Here's the drawing with two shaded views (mm, measured from the low corner). I have some questions. A direction names the side the tool comes from. Round coordinates to 2 decimals unless told otherwise and drop trailing zeros. Loops run counter-clockwise (first coordinate to the right, second up) from the corner with the lowest first, then second, coordinate; pieces in that order, holes last. Notation, with made-up numbers: (71, 51.5) -> (87, 51.5) arc R25 cw to (87, 88.5) -> close; hole circle Ø5 at (84.5, 22). An arc over 180 degrees is marked (long way). Write item = value, one per line.
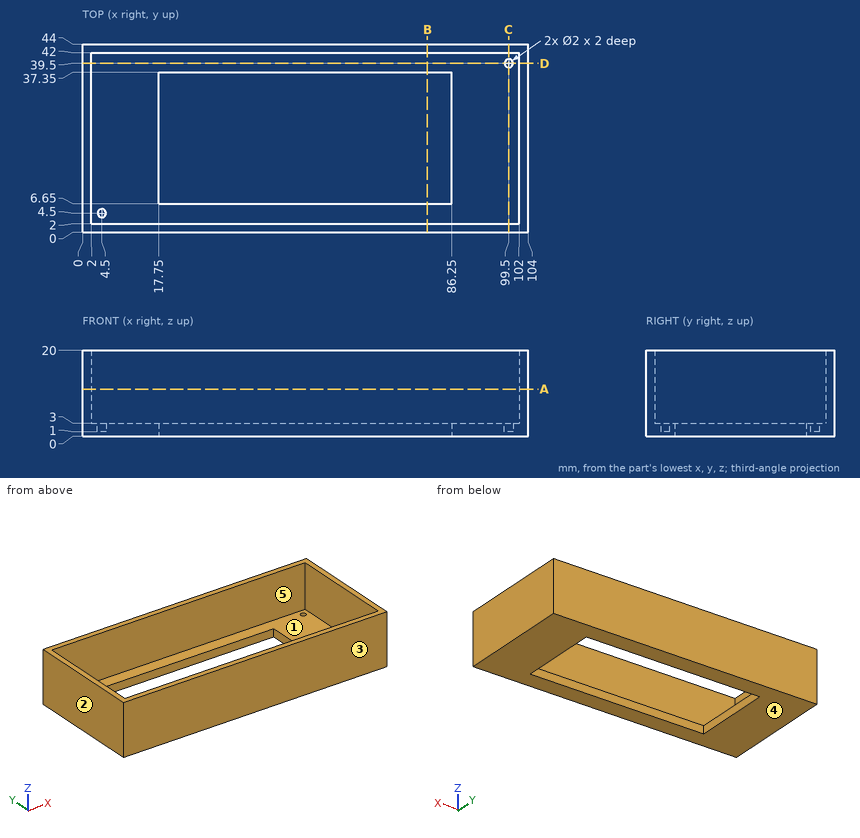
1. I need wall thicknesses on line 1 (Y direction, x = 66.5, z = 7); line 2 (Y direction, x = 4.5, z = 1.7); line 3 (X direction, y = 5.5, z = 13.5). Which ranges of each line are inside material? Lowest first, please. Write a range as [from, to].
Entries:
line_1 = [0, 2], [42, 44]
line_2 = [0, 3.5], [5.5, 44]
line_3 = [0, 2], [102, 104]
2. Suppose I cut it at C-C, the plane x = 99.5. List the corners of the cut face in (y, z) for me, and give its area (3 significant figures).
Entries:
outline = (0, 0) -> (44, 0) -> (44, 20) -> (42, 20) -> (42, 3) -> (40.5, 3) -> (40.5, 1) -> (38.5, 1) -> (38.5, 3) -> (2, 3) -> (2, 20) -> (0, 20) -> close
area = 196 mm²
3. We'd pull the mould along Y, two halves only. Please class the marked faces 3, 4 and 5: released by +Y, released by -Y, zero draft, split by the parting line, or undercut.
Entries:
face_3 = released by -Y
face_4 = zero draft
face_5 = undercut
4. Suppose I cut it at D-D, the plane y = 39.5. List the corners of the cut face in (x, z) for me.
Entries:
outline = (0, 0) -> (104, 0) -> (104, 20) -> (102, 20) -> (102, 3) -> (100.5, 3) -> (100.5, 1) -> (98.5, 1) -> (98.5, 3) -> (2, 3) -> (2, 20) -> (0, 20) -> close
5. Suppose I cut it at A-A, the plane z = 11. List the corners of the cut face in (x, y) for me, and give its area (3 significant figures).
Entries:
outline = (0, 0) -> (104, 0) -> (104, 44) -> (0, 44) -> close; hole (2, 2) -> (102, 2) -> (102, 42) -> (2, 42) -> close
area = 576 mm²
6. For the marked faces 1 and 2, which set-ups out of +Z, -Z, +X, -X, +Y, -Y let a thin tool reach every point of the face, with its end or its side?
Entries:
face_1 = +Z
face_2 = +Z, -Z, -X, +Y, -Y
7. Suppose I cut it at B-B, the plane x = 80.5. List the corners of the cut face in (y, z) for me.
Entries:
outline = (0, 0) -> (6.65, 0) -> (6.65, 3) -> (2, 3) -> (2, 20) -> (0, 20) -> close; (37.35, 0) -> (44, 0) -> (44, 20) -> (42, 20) -> (42, 3) -> (37.35, 3) -> close
8. I'm going to push flat-ended pins straight in: pin 1 (20 mm diameter, centred on x = 48.5, y = 14.5, fed in from +Z); pin 2 (1 mm diameter, centred on x = 99.5, y = 39.5, fed in from +Z). Where does each tip first touch, or does it pass through?
Entries:
pin_1 = 3
pin_2 = 1
